Autodesk Inventor part; units mm, degrees
ref_plane "YZ Plane" through (0, 0, 0) normal (1, 0, 0) x (0, 1, 0)
ref_plane "XZ Plane" through (0, 0, 0) normal (0, 1, 0) x (-1, 0, 0)
ref_plane "XY Plane" through (0, 0, 0) normal (0, 0, 1) x (1, 0, 0)
sketch "Sketch1" plane through (0, 0, 0) normal (0, 0, 1) x (1, 0, 0)
  line L0 (8.5, -5) -> (-8.5, -5)
  line L1 (-8.5, -5) -> (-8.5, 5)
  line L2 (-8.5, 5) -> (8.5, 5)
  line L3 (8.5, 5) -> (8.5, -5)
  line L4 (8.5, -5) -> (-8.5, 5) construction
  line L5 (-8.5, -5) -> (8.5, 5) construction
  point P0 (0, 0)
  dimension "d0" = 17
  dimension "d1" = 10
extrude "Extrusion1" add sketch "Sketch1" along normal blind 207.8
sketch "Sketch2" plane through (8.5, -5, 0) normal (1, 0, 0) x (0, 0, -1)
  line L0 (0, 10) -> (-207.8, 10)
  line L1 (-199.3, 10) -> (-199.3, 8)
  line L2 (-199.3, 8) -> (-202.8, 8)
  line L3 (-202.8, 8) -> (-202.8, 10)
  line L4 (-202.8, 10) -> (-207.8, 5)
  line L5 (-207.8, 5) -> (-202.8, 0)
  line L6 (-202.8, 0) -> (-202.8, 2)
  line L7 (-202.8, 2) -> (-199.3, 2)
  line L8 (-199.3, 2) -> (-199.3, 0)
  line L9 (0, 0) -> (-207.8, 0)
  line L10 (0, 10) -> (-207.8, 10)
  line L11 (-207.8, 0) -> (-207.8, 10)
  point P0 (0, 5)
  point P1 (-202.8, 0)
  point P2 (-202.8, 10)
  point P3 (-202.8, 10)
  dimension "d5" = 6
  dimension "d6" = 3.5
  dimension "d7" = 5
extrude "Extrusion2" cut sketch "Sketch2" against normal through all
fillet "Fillet1" radius 0.5 8 edges at (0, 5, 199.3) (0, 3, 199.3) (0, 3, 202.8) (0, 5, 202.8) (0, -5, 202.8) (0, -3, 202.8) (0, -3, 199.3) (0, -5, 199.3)
fillet "Fillet2" radius 2 1 edges at (0, 0, 207.8)
mirror "Mirror2" about plane through (0, 0, 0) normal (0, 0, -1)
sketch "Sketch3" plane through (-8.5, -5, 198.8) normal (0, 1, 0) x (1, 0, 0)
  point P0 (8.5, 198.8)
  point P1 (8.5, 71.8)
  point P2 (8.5, 325.8)
  dimension "d12" = 254
  dimension "d13" = 127
hole "Hole1" at (0, -5, 127) at (0, -5, -127) direction (0, 1, 0) diameter 9 end through all countersink diameter 17.3 countersink angle 90
properties part number "Support Rod" material "Aluminum 6061"
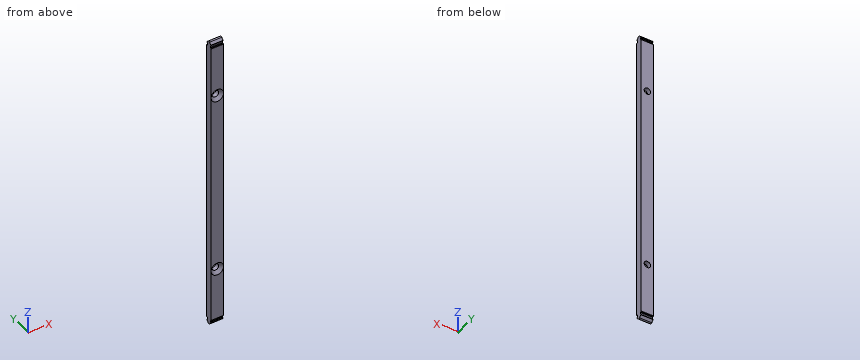
Design review of the part built by this model. Coordinates are the model's own, in mm. Coordinates: 2 decimals unless noted, no trailing zeros. Use a Markdown table: item, result.
(1) For P1, Ø0.5, axis at x = 3, y = 4, coming from the -Z side; P2, Ø2, axis at x = 1, z = 200.5, coming from the -Y side; P3, Ø0.8, axis at x = 2.5, z = 201, coming from the +Y side; P4, Ø8, axis at x = 0, z = 127, coming from the +Y side, all flat-tipped, find the tip position at first contact; note any pin that passes through.
Worked answers:
| item | result |
|---|---|
| P1 | stops at z = -204.05 |
| P2 | stops at y = -3.1 |
| P3 | stops at y = 3 |
| P4 | passes through |
(2) Wall thickness on probe 1 along X at (y, z) = (2, 127); probe 2 along X at (y, z) = (-3.75, -133.5); probe 3 along Z at (x, y) = (0, 0.45): over which ranges is each line inside the solid? List them lowest first.
Worked answers:
| item | result |
|---|---|
| probe 1 | x = -8.5 to -4.5, 4.5 to 8.5 |
| probe 2 | x = -8.5 to -3.54, 3.54 to 8.5 |
| probe 3 | z = -206.92 to -131.5, -122.5 to 122.5, 131.5 to 206.92 |
(3) Add section A-A (x = 0). Count the separate pieces of the cut face and the enclosed holes in it, then the cut area to 3 significant figures.
Worked answers:
| item | result |
|---|---|
| separate pieces | 3 |
| enclosed holes | 0 |
| area | 3,860 mm2 |
